Model file for the job. Use its own axes, mm. Round coordinates to 2 decimals unless told otherwise and drop trailing zeros. Order: outer loops, then holes, each group sorted by start corner. A loop starts at its lowest first (then second) coordinate and runs counter-clockwise, first axis right, second up. Notation, with made-up numbers: M 76.5,12.5 L 134.5,12.5 A10 ccw 134.5,27.5 Z; hole C 28,-29 d9. An arc over 180 degrees is marked long. Return JSON: item names as keys, results as strings. Group by question number.
Item 1: Slice it at C-C on z = -197. Write the cut outline in (x, y).
Item 2: Probe line 1 along Y through (x, z) = (0, -74); line 2 along Y through (x, z) = (5.75, -66.5). List the from-to ranges inside material, lowest first.
Item 3: Pin check, flat tips, straight feed: pin 1 Ø2 at (y, z) = (8.5, -144) entering from +X; pin 2 Ø10 at (x, z) = (-11, -79) entering from +Y; pin 3 Ø4 at (y, z) = (-11, -80.5) entering from -X; pin 4 Ø5 at (x, y) = (11.5, 8) entering from +Z. Stop position of each tip, or through.
Item 4: Slice it at A-A on y = 0. Write the cut outline in (x, z).
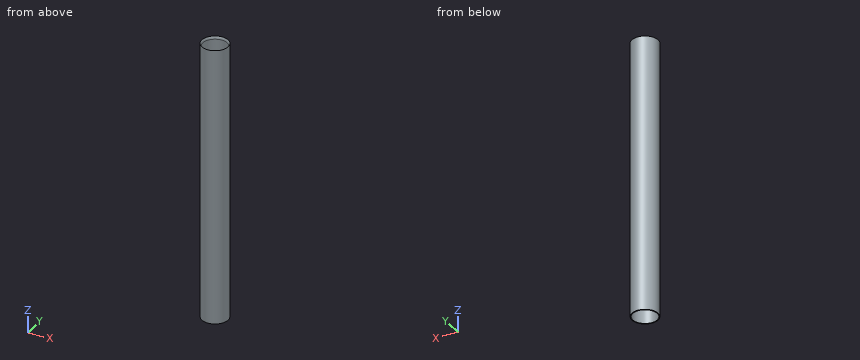
from build123d import *

# Parameters (mm, degrees)
SKETCH1_R           = 14.5
BOSS_EXTRUDE1_DEPTH = 304.8
SKETCH2_R           = 13.5
CUT_EXTRUDE1_DEPTH  = 304.8
FILLET3_R           = 5


with BuildPart() as part:
    # Sketch1 → Boss-Extrude1 (new body)
    with BuildSketch(Plane.XY):
        Circle(SKETCH1_R)
    extrude(amount=-BOSS_EXTRUDE1_DEPTH)

    # Sketch2 → Cut-Extrude1 (cut)
    with BuildSketch(Plane.XY):
        Circle(SKETCH2_R)
    extrude(amount=-CUT_EXTRUDE1_DEPTH, mode=Mode.SUBTRACT)

    # Fillet3
    # the kernel refuses this fillet: 5 mm, written as the material it takes off along each edge
    with BuildSketch(Plane(origin=(0, 0, 0), x_dir=(1, 0, 0), z_dir=(0, -1, 0))) as fillet3_piece_1:
        with BuildLine():
            CenterArc((18.5, -3), FILLET3_R, 143.130102354, 36.869897646)
            Line((13.5, -3), (13.4, -3))
            Line((13.4, -3), (13.4, 0))
            Line((13.4, 0), (13.5, 0.1))
            ThreePointArc((13.5, 0.1), (14, 0.1), (14.42, 0.06))
            Line((14.42, 0.06), (14.5, 0))
        make_face()
    revolve(axis=Axis((0, 0, 0), (0, 0, 1)), mode=Mode.SUBTRACT)


solid = part.part
Output values:
{
 "1": {"outline": "C 0,0 d29; hole C 0,0 d27"},
 "2": {"line 1": "-14.5 to -13.5, 13.5 to 14.5", "line 2": "-13.31 to -12.21, 12.21 to 13.31"},
 "3": {"pin 1": "x = 12.41", "pin 2": "y = 13.2", "pin 3": "x = -11.37", "pin 4": "z = 0"},
 "4": {"outline": "M -14.5,-304.8 L -13.5,-304.8 L -13.5,-3 A5 ccw -14.5,0 Z; M 13.5,-304.8 L 14.5,-304.8 L 14.5,0 A5 ccw 13.5,-3 Z"}
}
